Autodesk Inventor part; units mm, degrees
ref_plane "Work Plane2" through (3.35, 0, 0) normal (0, 0, -1) x (1, 0, 0)
ref_plane "YZ Plane" through (0, 0, 0) normal (1, 0, 0) x (0, 1, 0)
ref_plane "XZ Plane" through (0, 0, 0) normal (0, 1, 0) x (-1, 0, 0)
sketch "Sketch1" plane through (0, 0, 0) normal (0, 0, 1) x (1, 0, 0)
  line L0 (1.2, 0) -> (6, 0)
  line L1 (6, 0) -> (6, 1)
  line L2 (6, 1) -> (2, 1)
  line L3 (2, 1) -> (1.7546, 0.8773)
  line L4 (1.7546, 0.8773) -> (1.4071, 0.8773)
  line L5 (0, 1.9) -> (0, 0.95)
  line L6 (0, 0.95) -> (0.9455, 0.4786)
  line L7 (0.9455, 0.4786) -> (1.2, 0)
  line L8 (-1.2, 0) -> (7.2, 0)
  line L9 (0, -0.38) -> (0, 2.28)
  line L10 (0, 1.9) -> (0.1773, 1.9)
  line L11 (0.1773, 1.9) -> (1.0536, 1.0238)
  line L12 (2, 1) -> (1.0773, 1) construction
  arc A0 (1.0536, 1.0238) -> (1.4071, 0.8773) centre (1.4071, 1.3773) ccw
  point P0 (1.2, 0.8773)
  dimension "d1" = 4
  dimension "d2" = 2
  dimension "d3" = 1.7546
  dimension "d4" = 1.9
  dimension "d5" = 26.5
  dimension "d6" = 62
  dimension "d7" = 1.2
  dimension "d8" = 0.2454
  dimension "d12" = 3.8
  dimension "d13" = 45
  dimension "d15" = 6
  dimension "d24" = 1.2
  dimension "d93" = 0.5
revolve "Body" add sketch "Sketch1" angle 360 about axis through (1.2, 0, 0) along (1, 0, 0) contours L7 L6 L5 L10 L11 A0 L4 L3 L2 L1 L0
sketch "Sketch2" plane through (0, 0, 0) normal (-1, 0, 0) x (0, 0, 1)
  line L0 (0, 0.95) -> (0, 0) construction
  line L1 (0, 0) -> (0.95, 0) construction
  arc A0 (0.285, 0) -> (0, 0.285) centre (0, 0) ccw construction
  arc A1 (0.3325, 0) -> (0, 0.3325) centre (0, 0) ccw construction
  arc A2 (0.9373, 0.155) -> (0.155, 0.9373) centre (0, 0) ccw
  line L2 (0, 0) -> (0.6718, 0.6718) construction
  line L3 (0.155, 0.9373) -> (0.1646, 0.2889)
  line L4 (0.9373, 0.155) -> (0.2889, 0.1646)
  arc A3 (0.155, 0.9373) -> (0, 0.95) centre (0, 0) ccw
  arc A4 (0.95, 0) -> (0.9373, 0.155) centre (0, 0) ccw
  line L5 (0, -2.66) -> (0, 2.66)
  line L6 (-2.66, 0) -> (2.66, 0)
  arc A5 (0.155, -0.9373) -> (0.9373, -0.155) centre (0, 0) ccw
  line L7 (0.155, -0.9373) -> (0.1646, -0.2889)
  line L8 (0.9373, -0.155) -> (0.2889, -0.1646)
  arc A6 (0, -0.95) -> (0.155, -0.9373) centre (0, 0) ccw
  arc A7 (0.9373, -0.155) -> (0.95, 0) centre (0, 0) ccw
  arc A8 (-0.155, 0.9373) -> (-0.9373, 0.155) centre (0, 0) ccw
  line L9 (-0.155, 0.9373) -> (-0.1646, 0.2889)
  line L10 (-0.9373, 0.155) -> (-0.2889, 0.1646)
  arc A9 (0, 0.95) -> (-0.155, 0.9373) centre (0, 0) ccw
  arc A10 (-0.9373, 0.155) -> (-0.95, 0) centre (0, 0) ccw
  arc A11 (-0.155, -0.9373) -> (0, -0.95) centre (0, 0) ccw
  arc A12 (-0.9373, -0.155) -> (-0.155, -0.9373) centre (0, 0) ccw
  arc A13 (-0.95, 0) -> (-0.9373, -0.155) centre (0, 0) ccw
  line L11 (-0.9373, -0.155) -> (-0.2889, -0.1646)
  line L12 (-0.155, -0.9373) -> (-0.1646, -0.2889)
  arc A14 (0.1646, 0.2889) -> (0.2889, 0.1646) centre (0.2908, 0.2908) ccw
  arc A15 (0.2889, -0.1646) -> (0.1646, -0.2889) centre (0.2908, -0.2908) ccw
  arc A16 (-0.2889, 0.1646) -> (-0.1646, 0.2889) centre (-0.2908, 0.2908) ccw
  arc A17 (-0.1646, -0.2889) -> (-0.2889, -0.1646) centre (-0.2908, -0.2908) ccw
  point P0 (0.6718, -0.6718)
  point P1 (-0.6718, 0.6718)
  point P2 (-0.6718, -0.6718)
  dimension "d17" = 0.57
  dimension "d18" = 0.665
  dimension "d19" = 1.9
  dimension "d20" = 45
  dimension "d21" = 0.155
extrude "Slot" add sketch "Sketch2" against normal up to next draft 5 contours L4 A14 L3 A2 | A5 L7 A15 L8 | L9 A16 L10 A8 | A12 L11 A17 L12
fillet "Fillet1" radius 0.062 4 edges at (0, 0.95, 0) (0, 0, -0.95) (0, -0.95, 0) (0, 0, 0.95)
thread "Thread"
chamfer "Chamfer1" distance 0.2454 distance2 0.1227 1 edges at (6, -1, 0) measured on face at (6, 0.3275, -0.4215)
ref_plane "Work Plane2" through (3.35, 0, 0) normal (0, 0, -1) x (1, 0, 0)
equation "\"d1\" = GEL"
equation "\"d2\" = GD"
equation "\"d3\" = BDM"
equation "\"d4\" = SDM"
equation "\"d7\" = INTI"
equation "\"d8\" = GAL"
equation "\"d12\" = KOD"
equation "\"d13\" = 0.5 * SEWI"
equation "\"d15\" = NLG"
equation "\"d93\" = R"
equation "\"d17\" = 0.3 * SDM"
equation "\"d18\" = 0.35 * SDM"
equation "\"d19\" = SDM"
equation "\"d21\" = 0.5 * SBR"
equation "\"d23\" = 0.2 * SBR"
equation "\"d10\" = GEL"
equation "\"d25\" = -0.5 * SPD + 0.5 * GD"
equation "\"d26\" = 0.5 * GAL"
equation "\"NLG\" = 6"
equation "\"GEL\" = 4"
equation "\"GAL\" = 0.61345 * PTC"
equation "\"SPD\" = NND - 1.2269 * PTC"
equation "\"KOD\" = 3.8"
equation "\"KOH\" = 1.2"
equation "\"SBR\" = 0.31"
equation "\"INTI\" = 1.2"
equation "\"SDM\" = 1.9"
equation "\"GD\" = NND"
equation "\"BDM\" = NND - GAL"
equation "\"SEWI\" = 90deg"
equation "\"d9\" = SDM"
equation "\"R\" = 0.5"
equation "\"GUL\" = 0.61345 * PTC"
equation "\"TOA\" = 30deg"
equation "\"EPV\" = 2.2"
equation "\"THREADDIA\" = 2"
equation "\"PTC\" = 0.4"
equation "\"NND\" = 2"
equation "\"GD1\" = THREADDIA - 1.2269 * PTC"
properties part number "ISO 7046-1  - M2 x 6 - 4.8 - H" material "Steel"
Geometry check sheet. Reference: the model listing, model coordinates, mm. A direction names the side the tool comes from. Give positions to 0.01 mm unless a question says otherwise; leave off trailing zeros. Loops run counter-clockwise (first coordinate to the right, second up) from the corner with the lowest first, then second, coordinate; pieces in that order, holes last. Notation, with made-up numbers: M 57.5,84.5 L 62.5,84.5 A23 ccw 62.5,101.5 Z; hole C 26.25,-25 d10. An arc over 180 degrees is marked long. Answer as a JSON object with one key per item and string values. Group by question number.
Item 1: Material ranges on L1, parallel to Z at x = 1, y = 0.2; L2, parallel to Z at x = 0.5, y = 0.35; L3, parallel to X at y = 1.15, z = 1, recorded low to high.
Item 2: Gauge pin test, flat ends, axial feed: pin 1 (1.5 mm diameter, centred on x = 4.5, z = 1, fed in from +Y); pin 2 (1.5 mm diameter, centred on x = 1.5, y = 0, fed in from +Z); pin 3 (1.5 mm diameter, centred on x = 4.5, y = -1, fed in from -Z). Record the tip position at first contact, or that the pin passes through.
Item 3: Sectioned sample at A-A on x = 5.25. Record the boundary of the cut face in (y, z).
Item 4: Mould release check, pull along X, two halves, no side actions. Record for faces 3 (the cylindrical face through (1.58, 0.47, -0.74)), 4 (the flat face through (0, 0.4, -0.4)), 5 (the flat face through (6, 0, 0)): pulls with the +X half, pulls with the -X half, needs draft (parallel to the pull), parting line crosses it, or undercut.
Item 5: Access from +Z, -Z, +X, -X, +Y, -Y to the whole of each face (thin tool, end or side, straight path). Record for faces 1 (the conical face through (1.2, 0, 0)), 2 (the cylindrical face through (4, 0, 1)).
Findings below:
{
 "1": {"L1": "-1.06 to -0.1, 0.1 to 1.06", "L2": "-1.54 to -0.12, 0.12 to 1.54", "L3": "0 to 0.55"},
 "2": {"pin 1": "y = 0.97", "pin 2": "z = 1.33", "pin 3": "z = -0.97"},
 "3": {"outline": "C 0,0 d2"},
 "4": {"face 3": "undercut", "face 4": "pulls with the -X half", "face 5": "pulls with the +X half"},
 "5": {"face 1": "-X", "face 2": "+X"}
}
